Here's how the part is built. I have some questions about the finished solid (model axes, mm). Face numbers are marked on the shaded views. A direction names the side the tool comes from. Give positions to 0.01 mm unless a question says otherwise; leave off trailing zeros. Loops run counter-clockwise (first coordinate to the right, second up) from the corner with the lowest first, then second, coordinate; pieces in that order, holes last.
Q1. I need wall thicknesses on line 1 (Y direction, x = 0, z = 2.95); line 2 (Z direction, x = -18.5, y = -17); line 3 (Y direction, x = 0, z = 15). Which ranges of each line are inside material? Lowest first, please.
Q2. If we section it at D-D (x = 19.5): Please give me the cut outline in (y, z).
Q3. Will these pins go through, and if not, where does the flat tip stop? P1, Ø12, axis at y = -14.5, z = 7, coming from the +X side; P2, Ø8, axis at x = -6, z = 27, coming from the -Y side; P3, Ø12, axis at x = -5, y = 19.5, coming from the +Z side.
Q4. We'd pull the mould along X, two halves only. Please class the marked faces 4, 5 and 6: +X half, -X half, draft (parallel to the pull), parting line (faces both ways), or undercut.
Q5. If we section it at A-A (x = 0): Please give me the cut outline in (y, z).
Q6. For the marked faces 1, 2 and 3, which set-ups out of +Z, -Z, +X, -X, +Y, -Y let a thin tool reach every point of the face, with its end or its side?
Q7. If we section it at C-C (z = 12.5): Please give me the cut outline in (x, y), plus the area to 3 significant figures.
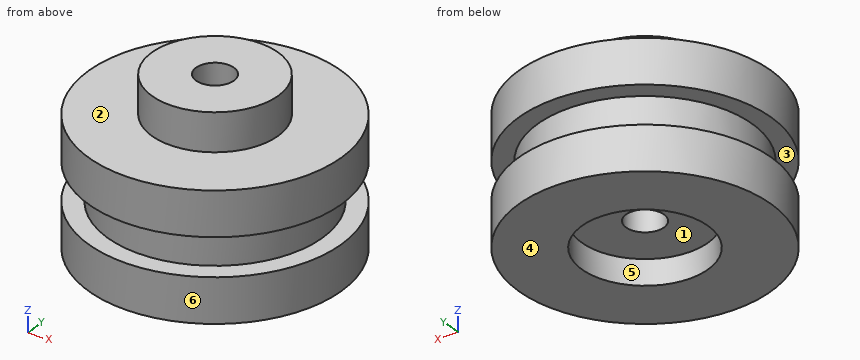
Autodesk Inventor part; units mm, degrees
ref_plane "Work Plane1" through (0, 0, 12.7) normal (0, 0, 1) x (1, 0, 0)
ref_plane "YZ Plane" through (0, 0, 0) normal (1, 0, 0) x (0, 1, 0)
ref_plane "XZ Plane" through (0, 0, 0) normal (0, 1, 0) x (-1, 0, 0)
sketch "Sketch1" plane through (0, 0, 0) normal (0, 0, 1) x (1, 0, 0)
  circle A0 centre (0, 0) radius 25.4
  dimension "d0" = 50.8
extrude "Extrusion1" add sketch "Sketch1" along normal blind 25.4
sketch "Sketch2" plane through (0, 0, 0) normal (0, 0, 1) x (1, 0, 0)
  point P0 (0, 0)
ref_plane "Work Plane1" through (0, 0, 12.7) normal (0, 0, 1) x (1, 0, 0)
sketch "Sketch4" plane through (0, 0, 12.7) normal (0, 0, 1) x (1, 0, 0)
  circle A0 centre (0, 0) radius 25.4
  circle A1 centre (0, 0) radius 21.59
  dimension "d7" = 50.8
  dimension "d8" = 43.18
extrude "Extrusion3" cut sketch "Sketch4" along normal mid plane 7.62
sketch "Sketch5" plane through (0, 0, 25.4) normal (0, 0, 1) x (1, 0, 0)
  circle A0 centre (0, 0) radius 12.7
  dimension "d11" = 25.4
extrude "Extrusion4" cut sketch "Sketch5" against normal blind 5.08
sketch "Sketch6" plane through (0, 0, 0) normal (0, 0, -1) x (-1, 0, 0)
  circle A0 centre (0, 0) radius 12.7
  dimension "d14" = 25.4
extrude "Extrusion5" cut sketch "Sketch6" against normal blind 5.08
sketch "Sketch7" plane through (0, 0, 20.32) normal (0, 0, 1) x (1, 0, 0)
  circle A0 centre (0, 0) radius 3.81
  dimension "d17" = 7.62
extrude "Extrusion6" cut sketch "Sketch7" along normal mid plane 127
sketch "Sketch8" plane through (0, 0, 20.32) normal (0, 0, 1) x (1, 0, 0)
  circle A0 centre (0, 0) radius 12.7
extrude "Extrusion7" add sketch "Sketch8" along normal blind 12.7
sketch "Sketch9" plane through (0, 0, 33.02) normal (0, 0, 1) x (1, 0, 0)
  circle A0 centre (0, 0) radius 3.81
  dimension "d22" = 7.62
extrude "Extrusion8" cut sketch "Sketch9" against normal blind 25.4
properties part number "Pulley"
Check sheet entries:
1. line 1: y = -25.4 to -12.7, 12.7 to 25.4
1. line 2: z = 0 to 8.89, 16.51 to 25.4
1. line 3: y = -21.59 to -3.81, 3.81 to 21.59
2. outline: (-16.28, 0) - (16.28, 0) - (16.28, 8.89) - (9.27, 8.89) - (9.27, 16.51) - (16.28, 16.51) - (16.28, 25.4) - (-16.28, 25.4) - (-16.28, 16.51) - (-9.27, 16.51) - (-9.27, 8.89) - (-16.28, 8.89) - close
3. P1: stops at x = 23.94
3. P2: stops at y = -25.29
3. P3: stops at z = 25.4
4. face 4: draft
4. face 5: undercut
4. face 6: parting line
5. outline: (-25.4, 0) - (-12.7, 0) - (-12.7, 5.08) - (-3.81, 5.08) - (-3.81, 33.02) - (-12.7, 33.02) - (-12.7, 25.4) - (-25.4, 25.4) - (-25.4, 16.51) - (-21.59, 16.51) - (-21.59, 8.89) - (-25.4, 8.89) - close; (3.81, 5.08) - (12.7, 5.08) - (12.7, 0) - (25.4, 0) - (25.4, 8.89) - (21.59, 8.89) - (21.59, 16.51) - (25.4, 16.51) - (25.4, 25.4) - (12.7, 25.4) - (12.7, 33.02) - (3.81, 33.02) - close
6. face 1: -Z
6. face 2: +Z
6. face 3: none
7. outline: circle Ø43.18 at (0, 0); hole circle Ø7.62 at (0, 0)
7. area: 1,420 mm2
